from build123d import *

# Parameters (mm, degrees)
F0_R     = 19.05
F1_DEPTH = 63.5
F2_R     = 5.5626
F3_DEPTH = 25.4


with BuildPart() as f1:
    # F0 (on Front) → F1 (new body)
    with BuildSketch(Plane.XZ):
        with BuildLine():
            Line((38.003319, 28.575), (0, 28.575))
            ThreePointArc((0, 28.575), (-19.473031, -20.912476), (28.502489, 2.034391))
            ThreePointArc((28.502489, 2.034391), (31.032493, 9.203532), (38.003319, 12.237521))
            Line((38.003319, 12.237521), (101.696681, 12.237521))
            Line((101.696681, 12.237521), (101.696681, 33.3502))
            Line((101.696681, 33.3502), (38.003319, 33.3502))
            Line((38.003319, 33.3502), (38.003319, 28.575))
        make_face()
        Circle(F0_R, mode=Mode.SUBTRACT)
    extrude(amount=F1_DEPTH)

    # F2 (on face) → F3 (cut)
    with BuildSketch(Plane.XY.offset(33.3502)):
        with BuildLine():
            ThreePointArc((90.449355, -20.722279), (96.8502, -31.75), (90.449355, -42.777721))
            Line((90.449355, -42.777721), (57.099155, -61.827721))
            ThreePointArc((57.099155, -61.827721), (54.058676, -63.074813), (50.8, -63.5))
            Line((50.8, -63.5), (101.696681, -63.5))
            Line((101.696681, -63.5), (101.696681, 0))
            Line((101.696681, 0), (50.8, 0))
            ThreePointArc((50.8, 0), (54.058676, -0.425187), (57.099155, -1.672279))
            Line((57.099155, -1.672279), (90.449355, -20.722279))
        make_face()
        with Locations((50.8, -50.8)):
            Circle(F2_R)
        with Locations((84.1502, -31.75)):
            Circle(F2_R)
        with Locations((50.8, -12.7)):
            Circle(F2_R)
    extrude(amount=-F3_DEPTH, mode=Mode.SUBTRACT)


solid = f1.part
Design review of the part built by this model. Coordinates are the model's own, in mm. A direction names the side the tool comes from. Round coordinates to 2 decimals unless told otherwise and drop trailing zeros. Write each loop counter-clockwise with the first axis right and the second up, starting at its lowest first coordinate (ties: lowest second). Pieces come first, ordered by that corner, then holes. Notation, with made-up numbers: (58, -27) -> (90, -27) arc R17 ccw to (90, 3) -> close; hole circle Ø11 at (7, -0.75). An arc over 180 degrees is marked (long way). One line per question, with ' | ' between items.
(1) Draft analysis for pull direction X (two halves, no side actions). For faces 4 (the cylindrical face through (-20.16, -31.31, -20.25)), 5 (the flat face through (19, -63.5, 3)), 6 (the cylindrical face through (53.79, -46.11, 22.94)), state which applies: released by +X, released by -X, zero draft, split by the parting line, or undercut.
Result sheet:
face 4: split by the parting line | face 5: zero draft | face 6: undercut
(2) Take a section at A-A, the plane y = -11. State the section outline as (x, z) points (3 decimals), and give its area (3 significant figures).
Result sheet:
outline: (0, 28.575) arc R28.575 ccw (long way) to (28.502, 2.034) arc R9.525 cw to (38.003, 12.238) -> (45.504, 12.238) -> (45.504, 33.35) -> (38.003, 33.35) -> (38.003, 28.575) -> close; (56.096, 12.238) -> (73.429, 12.238) -> (73.429, 33.35) -> (56.096, 33.35) -> close; hole circle Ø38.1 at (0, 0) | area: 2,300 mm2
(3) Take a section at B-B, the plane z = 0. State the section outline as (x, y) points (3 decimals), and give its area (3 significant figures).
Result sheet:
outline: (-28.575, -63.5) -> (-19.05, -63.5) -> (-19.05, 0) -> (-28.575, 0) -> close; (19.05, -63.5) -> (28.575, -63.5) -> (28.575, 0) -> (19.05, 0) -> close | area: 1,210 mm2
(4) Take a section at C-C, the plane x = 17.5. State the section outline as (y, z) points (3 decimals), and give its area (3 significant figures).
Result sheet:
outline: (-63.5, -22.589) -> (0, -22.589) -> (0, -7.527) -> (-63.5, -7.527) -> close; (-63.5, 7.527) -> (0, 7.527) -> (0, 28.575) -> (-63.5, 28.575) -> close | area: 2,290 mm2
(5) Wall thickness on line 1 (Y direction, x = 50.8, z = 18.25); line 2 (Z direction, x = 1, y = -57.5) (1 decimal); line 3 (Y direction, x = 50, z = 25): over which ranges is each line inside the solid? List them lowest first. Write a range as [from, to].
Result sheet:
line 1: [-63.5, -56.36], [-45.24, -18.26], [-7.14, 0] | line 2: [-28.6, -19], [19, 28.6] | line 3: [-63.5, -56.3], [-45.3, -18.2], [-7.2, 0]
(6) Insertion check: P1, Ø3, axis at x = 13.5, y = -56, coming from the +Z side (3 decimals); P2, Ø10, axis at x = 84.15, y = -31.75, coming from the +Z side; P3, Ø8, axis at x = 64.5, y = -20, coming from the -Z side; P4, Ø6, axis at y = -22, z = 23.5, coming from the +X side. Each pin has a flat end and moves straight along its axis. Give the tip position at first contact, or say it passes through.
Result sheet:
P1: z = 28.575 | P2: through | P3: z = 12.24 | P4: x = 94.91
(7) Take a section at D-D, the plane y = -59. State the section outline as (x, z) points (3 decimals).
Result sheet:
outline: (0, 28.575) arc R28.575 ccw (long way) to (28.502, 2.034) arc R9.525 cw to (38.003, 12.238) -> (62.05, 12.238) -> (62.05, 33.35) -> (38.003, 33.35) -> (38.003, 28.575) -> close; hole circle Ø38.1 at (0, 0)
(8) Machinability: for faces 1 (the flat face through (38.003, -31, 31)), 2 (the flat face through (60, -31, 12.238)), 3 (the cylindrical face through (53.79, -8.01, 22.94)), which of the approach directions +Z, -Z, +X, -X, +Y, -Y give a long, thin tool a straight path to every point of the face, cutting with its end or side? Answer none if there is none.
Result sheet:
face 1: +Z, -X, +Y, -Y | face 2: -Z, +X, +Y, -Y | face 3: +Z, -Z
